from build123d import *

# Parameters (mm, degrees)
SKETCH_1_R          = 51
SKETCH_1_R_2        = 23.5
EXTRUDE_1_DEPTH     = 8
SKETCH_2_R          = 31
SKETCH_2_R_2        = 27
EXTRUDE_2_DEPTH     = 5
CUT_EXTRUDE_1_REACH = 74.567
SKETCH_3_R          = 4.5


with BuildPart() as part:
    # 草图1 → 凸台-拉伸1 (new body)
    with BuildSketch(Plane.XY):
        Circle(SKETCH_1_R)
        Circle(SKETCH_1_R_2, mode=Mode.SUBTRACT)
    extrude(amount=EXTRUDE_1_DEPTH)

    # 草图2 → 凸台-拉伸2 (add)
    with BuildSketch(Plane.XY.offset(8)):
        Circle(SKETCH_2_R)
        Circle(SKETCH_2_R_2, mode=Mode.SUBTRACT)
    extrude(amount=EXTRUDE_2_DEPTH)

    # 草图3 → 切除-拉伸1 (cut, up to next)
    with BuildSketch(Plane.XY.offset(8), mode=Mode.PRIVATE) as cut_extrude_1_sk1:
        with Locations((41, 0)):
            Circle(SKETCH_3_R)
    cut_extrude_1_tool1 = extrude(cut_extrude_1_sk1.sketch, amount=-CUT_EXTRUDE_1_REACH, mode=Mode.PRIVATE) & part.part
    # 草图3 → 切除-拉伸1 (cut, up to next)
    with BuildSketch(Plane.XY.offset(8), mode=Mode.PRIVATE) as cut_extrude_1_sk2:
        with Locations((20.5, -35.507041555)):
            Circle(SKETCH_3_R)
    cut_extrude_1_tool2 = extrude(cut_extrude_1_sk2.sketch, amount=-CUT_EXTRUDE_1_REACH, mode=Mode.PRIVATE) & part.part
    # 草图3 → 切除-拉伸1 (cut, up to next)
    with BuildSketch(Plane.XY.offset(8), mode=Mode.PRIVATE) as cut_extrude_1_sk3:
        with Locations((-20.5, -35.507041555)):
            Circle(SKETCH_3_R)
    cut_extrude_1_tool3 = extrude(cut_extrude_1_sk3.sketch, amount=-CUT_EXTRUDE_1_REACH, mode=Mode.PRIVATE) & part.part
    # 草图3 → 切除-拉伸1 (cut, up to next)
    with BuildSketch(Plane.XY.offset(8), mode=Mode.PRIVATE) as cut_extrude_1_sk4:
        with Locations((-41, 0)):
            Circle(SKETCH_3_R)
    cut_extrude_1_tool4 = extrude(cut_extrude_1_sk4.sketch, amount=-CUT_EXTRUDE_1_REACH, mode=Mode.PRIVATE) & part.part
    # 草图3 → 切除-拉伸1 (cut, up to next)
    with BuildSketch(Plane.XY.offset(8), mode=Mode.PRIVATE) as cut_extrude_1_sk5:
        with Locations((-20.5, 35.507041555)):
            Circle(SKETCH_3_R)
    cut_extrude_1_tool5 = extrude(cut_extrude_1_sk5.sketch, amount=-CUT_EXTRUDE_1_REACH, mode=Mode.PRIVATE) & part.part
    # 草图3 → 切除-拉伸1 (cut, up to next)
    with BuildSketch(Plane.XY.offset(8), mode=Mode.PRIVATE) as cut_extrude_1_sk6:
        with Locations((20.5, 35.507041555)):
            Circle(SKETCH_3_R)
    cut_extrude_1_tool6 = extrude(cut_extrude_1_sk6.sketch, amount=-CUT_EXTRUDE_1_REACH, mode=Mode.PRIVATE) & part.part
    add(cut_extrude_1_tool1.solids().sort_by_distance((41, 0, 8))[0], mode=Mode.SUBTRACT)
    add(cut_extrude_1_tool2.solids().sort_by_distance((20.5, -35.507042, 8))[0], mode=Mode.SUBTRACT)
    add(cut_extrude_1_tool3.solids().sort_by_distance((-20.5, -35.507042, 8))[0], mode=Mode.SUBTRACT)
    add(cut_extrude_1_tool4.solids().sort_by_distance((-41, 0, 8))[0], mode=Mode.SUBTRACT)
    add(cut_extrude_1_tool5.solids().sort_by_distance((-20.5, 35.507042, 8))[0], mode=Mode.SUBTRACT)
    add(cut_extrude_1_tool6.solids().sort_by_distance((20.5, 35.507042, 8))[0], mode=Mode.SUBTRACT)


solid = part.part
Source: CAD feature listing. Evaluate the final solid. Frame: model axes, mm. A direction names the side the tool comes from. Round coordinates to 2 decimals unless told otherwise and drop trailing zeros. Write each loop counter-clockwise with the first axis right and the second up, starting at its lowest first coordinate (ties: lowest second). Pieces come first, ordered by that corner, then holes. Notation, with made-up numbers: M 22.5,-21 L 54.5,-21 A23 cw 54.5,-1 Z; hole C -23.75,70 d10. An arc over 180 degrees is marked long. One line per item, written item: value. Start each with the question number.
Item 1: Section query B-B (z = 1.75). Return the cut outline in (x, y).
Item 2: Pin query (flat end, axial travel): pin 1 (4 mm diameter, centred on y = 4.5, z = 9.5, fed in from +X); pin 2 (1.5 mm diameter, centred on y = -34.5, z = 6.5, fed in from -X); pin 3 (4 mm diameter, centred on y = -19, z = 9.5, fed in from -X). Return the tip coordinate at first contact, or that it passes through.
Item 3: Section query C-C (x = 20.5). Return the cut outline in (y, z), plus the area to 3 significant figures.
Item 4: Section query D-D (y = -25.5). Return the cut outline in (x, z), plus the area to 3 significant figures.
Item 5: Set-up query: faces 4 (the cylindrical face through (22.4, 7.1, 3.9)), 5 (the cylindrical face through (-5.85, -26.36, 10.46)). Return all of +Z, -Z, +X, -X, +Y, -Y with unobstructed straight access to the full face (end or side cutting, diameter ignored); none if empty.
Item 6: Ray query, L1, parallel to Y at x = 0, z = 11.55; L2, parallel to X at y = 33.5, z = 4.25; L3, parallel to Z at x = -41, y = 22. Return the intervals inside material, ascending. Write a range as from..to.
Item 7: Section query A-A (x = 0). Return the cut outline in (y, z), plus the area to 3 significant figures.
Item 8: Mould query, pull axis Y, two halves, no side actions, for faces 1 (the flat face through (-23, -22, 8)), 2 (the cylindrical face through (-24.071, -38.245, 4.056)), 3 (the cylindrical face through (-11.056, -49.787, 3.944)). Classes: pulls with the +Y half, pulls with the -Y half, needs draft (parallel to the pull), parting line crosses it, or undercut.
Result set:
1. outline: C 0,0 d102; hole C -41,0 d9; hole C -20.5,-35.51 d9; hole C -20.5,35.51 d9; hole C 0,0 d47; hole C 20.5,-35.51 d9; hole C 20.5,35.51 d9; hole C 41,0 d9
2. pin 1: stops at x = 50.9
2. pin 2: stops at x = -38.24
2. pin 3: stops at x = -47.84
3. outline: M -46.7,0 L -40.01,0 L -40.01,8 L -46.7,8 Z; M -31.01,0 L -11.49,0 L -11.49,8 L -17.57,8 L -17.57,13 L -23.25,13 L -23.25,8 L -31.01,8 Z; M 11.49,0 L 31.01,0 L 31.01,8 L 23.25,8 L 23.25,13 L 17.57,13 L 17.57,8 L 11.49,8 Z; M 40.01,0 L 46.7,0 L 46.7,8 L 40.01,8 Z
3. area: 476 mm²
4. outline: M -44.17,0 L 44.17,0 L 44.17,8 L 17.63,8 L 17.63,13 L 8.87,13 L 8.87,8 L -8.87,8 L -8.87,13 L -17.63,13 L -17.63,8 L -44.17,8 Z
4. area: 794 mm²
5. face 4: +Z, -Z
5. face 5: +Z
6. L1: y = -31..-27, 27..31
6. L2: x = -38.45..-24.53, -16.47..16.47, 24.53..38.45
6. L3: z = 0..8
7. outline: M -51,0 L -23.5,0 L -23.5,8 L -27,8 L -27,13 L -31,13 L -31,8 L -51,8 Z; M 23.5,0 L 51,0 L 51,8 L 31,8 L 31,13 L 27,13 L 27,8 L 23.5,8 Z
7. area: 480 mm²
8. face 1: needs draft
8. face 2: undercut
8. face 3: parting line crosses it
